Input: part model. Units: mm. Frame: model coordinates. A direction names the side the tool comes from. Coordinates: 2 decimals unless noted, no trailing zeros. Write each loop counter-clockwise with the first axis right and the second up, starting at its lowest first coordinate (ties: lowest second). Pieces come first, ordered by that corner, then holes. Notation, with made-up numbers: (68, -10.75) - (120, -10.75) arc R21 ccw to (120, 4.25) - close; hole circle Ø8 at (-33.75, -9.5). An arc over 180 degrees is marked (long way). One line per question, with ' | ' between items. Start each with the question number.
1) Reachability of faces 1 (the flat face through (39.65, 5.07, -9.86)), 2 (the flat face through (31, 10, -25)), 3 (the flat face through (0, 11, -24)) from +Z, -Z, +X, -X, +Y, -Y: full face, straight path, thin tool, end or side. Return the list, or none.
2) Section query C-C on x = 12. Return loops of the section in (y, z).
3) Line query: line 1 (X direction, y = 24.5, z = -38); line 2 (Y direction, x = 41.5, z = -38); line 3 (Y direction, x = 38, z = -18.5). Output: solid intervals per line, ascending.
4) Section query B-B on y = 18.5. Return loops of the section in (x, z), and give its area (3 significant figures).
5) First-contact query: P1, Ø6, axis at y = 19.5, z = -22.5, coming from the +X side; P2, Ø2, axis at x = 22, z = -31, coming from the +Y side. Flat tips, straight axial feed; report the tip coordinate or a pass-through.
6) Section query D-D on z = -34.5. Return loops of the section in (x, y).
7) Section query A-A on z = -9. Return loops of the section in (x, y).
```python
from build123d import *

# Parameters (mm, degrees)
SKETCH1_W           = 50
SKETCH1_H           = 40
BOSS_EXTRUDE4_DEPTH = 10
CUT_EXTRUDE1_DEPTH  = 20
SKETCH9_W           = 20
SKETCH9_H           = 40
BOSS_EXTRUDE5_DEPTH = 20
CUT_EXTRUDE3_DEPTH  = 20


with BuildPart() as part:
    # Sketch1 → Boss-Extrude4 (new body)
    with BuildSketch(Plane(origin=(0, 0, 0), x_dir=(1, 0, 0), z_dir=(0, 1, 0))):
        with Locations((25, 20)):
            Rectangle(SKETCH1_W, SKETCH1_H)
    extrude(amount=BOSS_EXTRUDE4_DEPTH)

    # Sketch8 → Cut-Extrude1 (cut)
    with BuildSketch(Plane.XY):
        Polygon((50, 0), (50, 10), (29.592919786, 10), align=None)
    extrude(amount=-CUT_EXTRUDE1_DEPTH, mode=Mode.SUBTRACT)

    # Sketch9 → Boss-Extrude5 (add)
    with BuildSketch(Plane(origin=(0, 10, 0), x_dir=(1, 0, 0), z_dir=(0, 1, 0))):
        with Locations((10, 20)):
            Rectangle(SKETCH9_W, SKETCH9_H)
    extrude(amount=BOSS_EXTRUDE5_DEPTH)

    # Sketch10 → Cut-Extrude3 (cut)
    with BuildSketch(Plane.ZY):
        Polygon((-40, 30), (0, 30), (0, 10), align=None)
    extrude(amount=-CUT_EXTRUDE3_DEPTH, mode=Mode.SUBTRACT)


solid = part.part
```
Answer key:
1) face 1: +Z, +X, +Y | face 2: +Z, -Z, +X, +Y | face 3: +Z, -Z, -X, +Y, -Y
2) outline: (0, -40) - (30, -40) - (10, 0) - (0, 0) - close
3) line 1: 0 to 20 | line 2: 0 to 10 | line 3: 0 to 5.88
4) outline: (0, -40) - (20, -40) - (20, -17) - (0, -17) - close | area: 460 mm²
5) P1: x = 20 | P2: y = 10
6) outline: (0, 0) - (50, 0) - (50, 10) - (20, 10) - (20, 27.25) - (0, 27.25) - close
7) outline: (0, 0) - (50, 0) - (29.59, 10) - (20, 10) - (20, 14.5) - (0, 14.5) - close
